```python
from build123d import *

# Parameters (mm, degrees)
BOSS_EXTRUDE2_DEPTH                      = 45
SHELL1_T                                 = 5
CUT_EXTRUDE1_REACH                       = 47
SKETCH7_W                                = 35
SKETCH7_H                                = 30
CUT_EXTRUDE2_DEPTH                       = 46
CUT_EXTRUDE5_REACH                       = 49.5
SKETCH9_W                                = 20
SKETCH9_H                                = 35
CBORE_FOR_M16_HEX_HEAD_BOLT1_D           = 11
CBORE_FOR_M16_HEX_HEAD_BOLT1_DEPTH       = 5
CBORE_FOR_M16_HEX_HEAD_BOLT1_CBORE_D     = 16
CBORE_FOR_M16_HEX_HEAD_BOLT1_CBORE_DEPTH = 3
CBORE_FOR_M16_HEX_HEAD_BOLT1_TIP         = 3.304733405
CUT_EXTRUDE6_REACH                       = 49.5
SKETCH11_R                               = 2
FILLET1_R                                = 3
CUT_EXTRUDE10_REACH                      = 47
SKETCH15_R                               = 10
CBORE_FOR_M5_HEX_HEAD_BOLT1_D            = 5
CBORE_FOR_M5_HEX_HEAD_BOLT1_CBORE_D      = 10
CBORE_FOR_M5_HEX_HEAD_BOLT1_CBORE_DEPTH  = 2


with BuildPart() as part:
    # Sketch5 → Boss-Extrude2 (new body)
    with BuildSketch(Plane.XY):
        Polygon((-15, -20), (15, -20), (22.5, -12.5), (22.5, 27.5), (-22.5, 27.5), (-22.5, -12.5), align=None)
    extrude(amount=-BOSS_EXTRUDE2_DEPTH)

    # Shell1 (no face opened: a closed hollow body)
    add(offset(amount=-SHELL1_T, mode=Mode.PRIVATE), mode=Mode.SUBTRACT)

    # Sketch6 → Cut-Extrude1 (cut, up to next)
    with BuildSketch(Plane(origin=(0, 0, -45), x_dir=(-1, 0, 0), z_dir=(0, 0, -1)), mode=Mode.PRIVATE) as cut_extrude1_sk1:
        Polygon((12.928932188, -15), (17.5, -10.428932188), (17.5, 22.5), (-17.5, 22.5), (-17.5, -10.428932188), (-12.928932188, -15), align=None)
    cut_extrude1_tool1 = extrude(cut_extrude1_sk1.sketch, amount=-CUT_EXTRUDE1_REACH, mode=Mode.PRIVATE) & part.part
    add(cut_extrude1_tool1.solids().sort_by_distance((0, 4.028675, -45))[0], mode=Mode.SUBTRACT)

    # Sketch7 → Cut-Extrude2 (cut, through all)
    with BuildSketch(Plane(origin=(22.5, 0, 0), x_dir=(0, 0, -1), z_dir=(1, 0, 0))):
        with Locations((22.5, 7.5)):
            Rectangle(SKETCH7_W, SKETCH7_H)
    extrude(amount=-CUT_EXTRUDE2_DEPTH, mode=Mode.SUBTRACT)

    # Sketch9 → Cut-Extrude5 (cut, up to next)
    with BuildSketch(Plane.XZ.offset(20), mode=Mode.PRIVATE) as cut_extrude5_sk1:
        with Locations((0, -22.5)):
            Rectangle(SKETCH9_W, SKETCH9_H)
    cut_extrude5_tool1 = extrude(cut_extrude5_sk1.sketch, amount=-CUT_EXTRUDE5_REACH, mode=Mode.PRIVATE) & part.part
    add(cut_extrude5_tool1.solids().sort_by_distance((0, -20, -22.5))[0], mode=Mode.SUBTRACT)

    # Sketch1 → Revolve1 (revolve)
    with BuildSketch(Plane(origin=(0, 0, 0), x_dir=(0, 0, -1), z_dir=(1, 0, 0)), mode=Mode.PRIVATE) as revolve1_sk:
        with BuildLine():
            Line((0, 10), (-35, 10))
            ThreePointArc((-35, 10), (-35.944911183, 10.672673165), (-35.618589574, 11.785714286))
            ThreePointArc((-35.618589574, 11.785714286), (-31.249648492, 14.173667738), (-26.339745962, 15))
            Line((-26.339745962, 15), (0, 15))
            Line((0, 15), (0, 10))
        make_face()
    revolve(revolve1_sk.sketch.rotate(Axis((0, 0, 0), (0, 0, 1)), 90), axis=Axis((0, 0, 0), (0, 0, 1)))  # turned: the seam where the file's is

    # Sketch10 → Revolve2 (revolve)
    with BuildSketch(Plane(origin=(0, 0, 0), x_dir=(0, 0, -1), z_dir=(1, 0, 0))):
        with BuildLine():
            Line((38.5, 27.5), (38.5, 29.5))
            ThreePointArc((38.5, 29.5), (39.5, 30.5), (40.5, 29.5))
            Line((40.5, 29.5), (40.5, 27.5))
            Line((40.5, 27.5), (38.5, 27.5))
        make_face()
    revolve(axis=Axis((0, 27.5, -22.5), (0, 1, 0)))

    # CBORE for M16 Hex Head Bolt1
    with Locations(Plane(origin=(0, 27.5, 0), x_dir=(1, 0, 0), z_dir=(0, 1, 0))):
        with Locations((0, 22.5)):
            CounterBoreHole(CBORE_FOR_M16_HEX_HEAD_BOLT1_D / 2, CBORE_FOR_M16_HEX_HEAD_BOLT1_CBORE_D / 2, CBORE_FOR_M16_HEX_HEAD_BOLT1_CBORE_DEPTH, depth=CBORE_FOR_M16_HEX_HEAD_BOLT1_DEPTH)
            with Locations((0, 0, -(CBORE_FOR_M16_HEX_HEAD_BOLT1_DEPTH + CBORE_FOR_M16_HEX_HEAD_BOLT1_TIP / 2))):  # 118° drill point
                Cone(0, CBORE_FOR_M16_HEX_HEAD_BOLT1_D / 2, CBORE_FOR_M16_HEX_HEAD_BOLT1_TIP, mode=Mode.SUBTRACT)

    # Sketch11 → Cut-Extrude6 (cut, up to next)
    with BuildSketch(Plane(origin=(0, 27.5, 0), x_dir=(1, 0, 0), z_dir=(0, 1, 0)), mode=Mode.PRIVATE) as cut_extrude6_sk1:
        with Locations(Location((12, 22.5, 0), (0, 0, 270))):  # turned: the seam where the file's is
            Circle(SKETCH11_R)
    cut_extrude6_tool1 = extrude(cut_extrude6_sk1.sketch, amount=-CUT_EXTRUDE6_REACH, mode=Mode.PRIVATE) & part.part
    add(cut_extrude6_tool1.solids().sort_by_distance((12, 27.5, -22.5))[0], mode=Mode.SUBTRACT)
    # Sketch11 → Cut-Extrude6 (cut, up to next)
    with BuildSketch(Plane(origin=(0, 27.5, 0), x_dir=(1, 0, 0), z_dir=(0, 1, 0)), mode=Mode.PRIVATE) as cut_extrude6_sk2:
        with Locations(Location((0, 10.5, 0), (0, 0, 270))):  # turned: the seam where the file's is
            Circle(SKETCH11_R)
    cut_extrude6_tool2 = extrude(cut_extrude6_sk2.sketch, amount=-CUT_EXTRUDE6_REACH, mode=Mode.PRIVATE) & part.part
    add(cut_extrude6_tool2.solids().sort_by_distance((0, 27.5, -10.5))[0], mode=Mode.SUBTRACT)
    # Sketch11 → Cut-Extrude6 (cut, up to next)
    with BuildSketch(Plane(origin=(0, 27.5, 0), x_dir=(1, 0, 0), z_dir=(0, 1, 0)), mode=Mode.PRIVATE) as cut_extrude6_sk3:
        with Locations(Location((-12, 22.5, 0), (0, 0, 270))):  # turned: the seam where the file's is
            Circle(SKETCH11_R)
    cut_extrude6_tool3 = extrude(cut_extrude6_sk3.sketch, amount=-CUT_EXTRUDE6_REACH, mode=Mode.PRIVATE) & part.part
    add(cut_extrude6_tool3.solids().sort_by_distance((-12, 27.5, -22.5))[0], mode=Mode.SUBTRACT)
    # Sketch11 → Cut-Extrude6 (cut, up to next)
    with BuildSketch(Plane(origin=(0, 27.5, 0), x_dir=(1, 0, 0), z_dir=(0, 1, 0)), mode=Mode.PRIVATE) as cut_extrude6_sk4:
        with Locations(Location((0, 34.5, 0), (0, 0, 270))):  # turned: the seam where the file's is
            Circle(SKETCH11_R)
    cut_extrude6_tool4 = extrude(cut_extrude6_sk4.sketch, amount=-CUT_EXTRUDE6_REACH, mode=Mode.PRIVATE) & part.part
    add(cut_extrude6_tool4.solids().sort_by_distance((0, 27.5, -34.5))[0], mode=Mode.SUBTRACT)

    # Fillet1
    fillet1_edges = [part.edges().sort_by_distance(p)[0] for p in [
        (15, 0, 0),
    ]]
    fillet(fillet1_edges, radius=FILLET1_R)

    # Sketch15 → Cut-Extrude10 (cut, up to next)
    with BuildSketch(Plane.XY, mode=Mode.PRIVATE) as cut_extrude10_sk1:
        with Locations(Location((0, 0, 0), (0, 0, 180))):  # turned: the seam where the file's is
            Circle(SKETCH15_R)
    cut_extrude10_tool1 = extrude(cut_extrude10_sk1.sketch, amount=-CUT_EXTRUDE10_REACH, mode=Mode.PRIVATE) & part.part
    add(cut_extrude10_tool1.solids().sort_by_distance((0, 0, 0))[0], mode=Mode.SUBTRACT)

    # CBORE for M5 Hex Head Bolt1 (through all)
    with Locations(Plane(origin=(15, 0, 0), x_dir=(0, 0, -1), z_dir=(1, 0, 0))):
        with Locations((-15, 0)):
            cbore_for_m5_hex_head_bolt1 = CounterBoreHole(CBORE_FOR_M5_HEX_HEAD_BOLT1_D / 2, CBORE_FOR_M5_HEX_HEAD_BOLT1_CBORE_D / 2, CBORE_FOR_M5_HEX_HEAD_BOLT1_CBORE_DEPTH)

    # Mirror1: CBORE for M5 Hex Head Bolt1 across plane
    add(cbore_for_m5_hex_head_bolt1.mirror(Plane(origin=(0, 0, 0), x_dir=(0, 0, 1), z_dir=(1, 0, 0))), mode=Mode.SUBTRACT)


solid = part.part
```
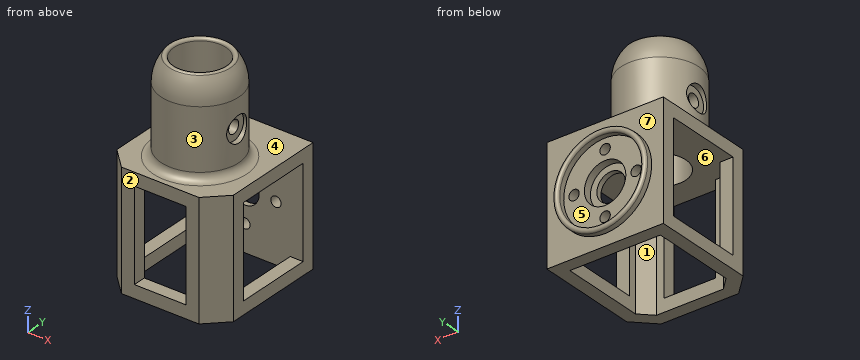
Geometry check sheet. Reference: the model listing, model coordinates, mm. Face numbers are marked on the shaded views. A direction names the side the tool comes from. Coordinates: 2 decimals unless noted, no trailing zeros. Order: outer loops, then holes, each group sorted by start corner. A loop starts at its lowest first (then second) coordinate and runs counter-clockwise, first axis right, second up.
Item 1: Tool access check on the marked faces 1, 2 and 3. Record the directions out of +Z, -Z, +X, -X, +Y, -Y that give a thin tool (end or side, any length) a straight path to the whole face; none if there is none.
Item 2: Mould release check, pull along Z, two halves, no side actions. Record for the marked faces 4, 5, 6 and 7: released by +Z, released by -Z, zero draft, split by the parting line, or undercut.
Item 3: Section check A-A (z = -22.5). Count the separate pieces of the cut face and the enclosed holes in it, plus the area to 3 significant figures.
Item 4: Section check C-C (z = 15). Enter the section's corners in (x, y), plus the area to 3 significant figures.
Item 5: Depth check by flat-ended pin: pin 1 (10 mm diameter, centred on x = 0, z = -22.5, fed in from +Y); pin 2 (17.5 mm diameter, centred on x = -1, z = -22.5, fed in from +Y); pin 3 (3 mm diameter, centred on y = 1.5, z = 13.5, fed in from -X); pin 4 (4 mm diameter, centred on x = -3, z = -26, fed in from -Y). Enter the tip coordinate at first touch or a pass-through.
Item 6: Scan lines: line 1 along Y through (x, z) = (0, 5); line 2 along Z through (x, y) = (20.5, 4); line 3 along Y through (x, z) = (3, -11). Record each from-to range of solid material in increasing order.
Check sheet entries:
1. face 1: -Z
1. face 2: +Z, -Z, +X, -X, -Y
1. face 3: +Z
2. face 4: released by +Z
2. face 5: undercut
2. face 6: undercut
2. face 7: zero draft
3. separate pieces: 6
3. enclosed holes: 0
3. area: 291 mm2
4. outline: (-14.14, -5) arc R15 ccw to (14.14, -5) - (13, -5) - (13, -2.5) - (9.68, -2.5) arc R10 cw to (-9.68, -2.5) - (-13, -2.5) - (-13, -5) - close; (-14.14, 5) - (-13, 5) - (-13, 2.5) - (-9.68, 2.5) arc R10 cw to (9.68, 2.5) - (13, 2.5) - (13, 5) - (14.14, 5) arc R15 ccw to start
4. area: 327 mm2
5. pin 1: passes through
5. pin 2: stops at y = 27.5
5. pin 3: stops at x = -13
5. pin 4: stops at y = 22.5
6. line 1: y = -15 to -10, 10 to 15
6. line 2: z = -45 to -40, -5 to 0
6. line 3: y = 22.5 to 27.5
